```python
from build123d import *

# Parameters (mm, degrees)
SKETCH1_W           = 76.2
SKETCH1_H           = 76.2
BOSS_EXTRUDE1_DEPTH = 2.9718
SKETCH2_W           = 25.4
SKETCH2_H           = 2.9718
SKETCH2_W_2         = 12.7
SKETCH2_W_3         = 2.9718
SKETCH2_H_2         = 12.7
SKETCH2_H_3         = 25.4
SKETCH2_R           = 1.4224
CUT_EXTRUDE1_DEPTH  = 54.963428313


with BuildPart() as part:
    # Sketch1 → Boss-Extrude1 (new body)
    with BuildSketch(Plane(origin=(0, 0, 0), x_dir=(1, 0, 0), z_dir=(0, 1, 0))):
        Rectangle(SKETCH1_W, SKETCH1_H)
    extrude(amount=BOSS_EXTRUDE1_DEPTH)

    # Sketch2 → Cut-Extrude1 (cut, through all)
    with BuildSketch(Plane(origin=(0, 2.9718, 0), x_dir=(1, 0, 0), z_dir=(0, 1, 0))):
        with Locations((-25.4, 36.6141)):
            Rectangle(SKETCH2_W, SKETCH2_H)
        with Locations((31.75, 36.6141)):
            Rectangle(SKETCH2_W_2, SKETCH2_H)
        with Locations((36.6141, 31.75)):
            Rectangle(SKETCH2_W_3, SKETCH2_H_2)
        with Locations((36.6141, -25.4)):
            Rectangle(SKETCH2_W_3, SKETCH2_H_3)
        with Locations(Location((36.6141, 6.35, 0), (0, 0, 270))):
            Circle(SKETCH2_R)
        with Locations(Location((6.35, 36.6141, 0), (0, 0, 270))):
            Circle(SKETCH2_R)
        with Locations((31.75, -36.6141)):
            Rectangle(SKETCH2_W_2, SKETCH2_H)
        with Locations(Location((6.35, -36.6141, 0), (0, 0, 270))):
            Circle(SKETCH2_R)
        with Locations((-25.4, -36.6141)):
            Rectangle(SKETCH2_W, SKETCH2_H)
    extrude(amount=-CUT_EXTRUDE1_DEPTH, mode=Mode.SUBTRACT)


solid = part.part
```
Here's how the part is built. I have some questions about the finished solid (model axes, mm). A direction names the side the tool comes from. Round coordinates to 2 decimals unless told otherwise and drop trailing zeros. Order: outer loops, then holes, each group sorted by start corner. A loop starts at its lowest first (then second) coordinate and runs counter-clockwise, first axis right, second up. Notation, with made-up numbers: M -8,74.25 L 11,74.25 A25 ccw 11,104.25 Z; hole C 70.5,-7 d11. An arc over 180 degrees is marked long. One line per question, with ' | ' between items.
1) I want a section at D-D, the plane z = -29.5. Write out the boundary of the cut face in (x, y).
Working result:
outline: M -38.1,0 L 35.13,0 L 35.13,2.97 L -38.1,2.97 Z
2) I want a section at B-B, the plane x = 6.35. Write out the boundary of the cut face in (y, z).
Working result:
outline: M 0,-38.1 L 2.97,-38.1 L 2.97,-38.04 L 0,-38.04 Z; M 0,-35.19 L 2.97,-35.19 L 2.97,35.19 L 0,35.19 Z; M 0,38.04 L 2.97,38.04 L 2.97,38.1 L 0,38.1 Z
3) I want a section at A-A, the plane z = -6.35. Write out the boundary of the cut face in (x, y).
Working result:
outline: M -38.1,0 L 35.19,0 L 35.19,2.97 L -38.1,2.97 Z; M 38.04,0 L 38.1,0 L 38.1,2.97 L 38.04,2.97 Z
4) For pin 1 Ø1.5 at (y, z) = (1, -37.5) entering from +X; pin 2 Ø0.9 at (x, y) = (30, 1.5) entering from -Z; pin 3 Ø0.9 at (x, y) = (36, 1) entering from -Z, each with a flat end and sliding along its axis, tell me the tip position at first contact or that it passes through.
Working result:
pin 1: x = 25.4 | pin 2: z = -35.13 | pin 3: z = -25.4
5) I need wall thicknesses on line 1 along Z through (x, y) = (5.5, 1.65); line 2 along X through (y, z) = (2.7, 28.5); line 3 along Z through (x, y) = (35, 2.6). Which ranges of each line are inside material? Lowest first, please.
Working result:
line 1: -38.1 to -37.75, -35.47 to 35.47, 37.75 to 38.1 | line 2: -38.1 to 35.13 | line 3: -35.13 to 35.13
6) I want a section at C-C, the plane y = 1.65. Write out the boundary of the cut face in (x, z).
Working result:
outline: M -38.1,-35.13 L -12.7,-35.13 L -12.7,-38.1 L 25.4,-38.1 L 25.4,-35.13 L 35.13,-35.13 L 35.13,-25.4 L 38.1,-25.4 L 38.1,12.7 L 35.13,12.7 L 35.13,35.13 L 25.4,35.13 L 25.4,38.1 L -12.7,38.1 L -12.7,35.13 L -38.1,35.13 Z; hole C 6.35,-36.61 d2.84; hole C 6.35,36.61 d2.84; hole C 36.61,-6.35 d2.84
7) If we mould it in two halves opening along Z, with no side actions, what happens to faces 6 (the face through (37.575, 1.507, -7.398)), 7 (the face through (-12.7, 2, 37)), 8 (the face through (37, 2, 12.7))? For each: +Z half, -Z half, draft (parallel to the pull), parting line (faces both ways), or undercut.
Working result:
face 6: undercut | face 7: draft | face 8: +Z half
8) For faces 1 (the face through (-12.7, 2, -37)), 2 (the face through (-26, 2, 35.128)), 3 (the face through (30, 2, -35.128)), 4 (the face through (-1, 2.972, -1)), 5 (the face through (30, 2, 35.128)), which set-ups out of +Z, -Z, +X, -X, +Y, -Y let a thin tool reach every point of the face, with its end or its side?
Working result:
face 1: -Z, -X, +Y, -Y | face 2: +Z, -X, +Y, -Y | face 3: -Z, +X, +Y, -Y | face 4: +Z, -Z, +X, -X, +Y | face 5: +Z, +X, +Y, -Y
